Part model, mm, in its own coordinate system. A direction names the side the tool comes from. Round coordinates to 2 decimals unless told otherwise and drop trailing zeros. Write each loop counter-clockwise with the first axis right and the second up, starting at its lowest first coordinate (ties: lowest second). Pieces come first, ordered by that corner, then holes.
```python
from build123d import *

# Parameters (mm, degrees)
SKETCH_1_W      = 20
SKETCH_1_H      = 18
SKETCH_1_R      = 1.5
EXTRUDE_1_DEPTH = 1.6
SKETCH_2_W      = 7.6
SKETCH_2_H      = 9
EXTRUDE_2_DEPTH = 4


with BuildPart() as part:
    # 草图1 → 凸台-拉伸1 (new body)
    with BuildSketch(Plane(origin=(0, 0, 0), x_dir=(1, 0, 0), z_dir=(0, 1, 0))):
        with Locations((10, 9)):
            Rectangle(SKETCH_1_W, SKETCH_1_H)
        with Locations(Location((2.5, 5, 0), (0, 0, 270))):
            Circle(SKETCH_1_R, mode=Mode.SUBTRACT)
        with Locations(Location((17.5, 5, 0), (0, 0, 90))):
            Circle(SKETCH_1_R, mode=Mode.SUBTRACT)
    extrude(amount=EXTRUDE_1_DEPTH)

    # 草图2 → 凸台-拉伸2 (add)
    with BuildSketch(Plane(origin=(0, 1.6, 0), x_dir=(1, 0, 0), z_dir=(0, 1, 0))):
        with Locations((10, 13.5)):
            Rectangle(SKETCH_2_W, SKETCH_2_H)
    extrude(amount=EXTRUDE_2_DEPTH)


solid = part.part
```
Q1. Cut at B-B on x = 1.5. Write the cut outline in (y, z).
Values follow:
outline: (0, -18) - (1.6, -18) - (1.6, -6.12) - (0, -6.12) - close; (0, -3.88) - (1.6, -3.88) - (1.6, 0) - (0, 0) - close
Q2. Cut at A-A on z = -5. Write the cut outline in (x, y).
Values follow:
outline: (0, 0) - (1, 0) - (1, 1.6) - (0, 1.6) - close; (4, 0) - (16, 0) - (16, 1.6) - (4, 1.6) - close; (19, 0) - (20, 0) - (20, 1.6) - (19, 1.6) - close
Q3. Cut at D-D on z = -10. Write the cut outline in (x, y), plus the area to 3 significant figures.
Values follow:
outline: (0, 0) - (20, 0) - (20, 1.6) - (13.8, 1.6) - (13.8, 5.6) - (6.2, 5.6) - (6.2, 1.6) - (0, 1.6) - close
area: 62.4 mm2
Q4. Wall check: L1, parallel to X at y = 0.6, z = -5; L2, parallel to Z at x = 17.5, y = 0.65; L3, parallel to X at y = 1.1, z = -5.75. Give the ranges that are in metal, low to high.
Values follow:
L1: x = 0 to 1, 4 to 16, 19 to 20
L2: z = -18 to -6.5, -3.5 to 0
L3: x = 0 to 1.2, 3.8 to 16.2, 18.8 to 20
Q5. Which spindle directions (+Z, -Z, +X, -X, +Y, -Y) get a long thin tool onto all of the face, cutting with end or side? Do faces 1 (the flat face through (10, 4, -9)), 2 (the flat face through (6.2, 4, -13)), 3 (the flat face through (13.8, 4, -13)), 4 (the flat face through (10, 5.6, -14)). Say none if no direction does.
Values follow:
face 1: +Z, +X, -X, +Y
face 2: +Z, -Z, -X, +Y
face 3: +Z, -Z, +X, +Y
face 4: +Z, -Z, +X, -X, +Y
Q6. Drop flat-ended pins along their axis: pin 1 (1 mm diameter, centred on y = 4, z = -7.5, fed in from -X); pin 2 (3.5 mm diameter, centred on x = 2.5, z = -5, fed in from -Y); pin 3 (2 mm diameter, centred on y = 4, z = -13, fed in from +X); pin 4 (3 mm diameter, centred on y = 4.5, z = -12, fed in from -X). Give the stop position or say it passes through.
Values follow:
pin 1: passes through
pin 2: stops at y = 0
pin 3: stops at x = 13.8
pin 4: stops at x = 6.2
Q7. Cut at C-C on y = 0.6. Write the cut outline in (x, z), plus the area to 3 significant figures.
Values follow:
outline: (0, -18) - (20, -18) - (20, 0) - (0, 0) - close; hole circle Ø3 at (2.5, -5); hole circle Ø3 at (17.5, -5)
area: 346 mm2
Q8. Mould opens along X. For faces 5 (the cylindrical face through (16.235, 0.789, -5.806)), 6 (the flat face through (10, 1, 0)), 7 (the flat face through (0, 1, -9)) say: +X half, -X half, draft (parallel to the pull), parting line (faces both ways), or undercut.
Values follow:
face 5: undercut
face 6: draft
face 7: -X half
